```python
from build123d import *

# Parameters (mm, degrees)
SKETCH3_W           = 10.7
SKETCH3_H           = 10.7
BOSS_EXTRUDE2_DEPTH = 2.41
SKETCH5_R           = 1.25
BOSS_EXTRUDE3_DEPTH = 1.5875


with BuildPart() as part:
    # Sketch3 → Boss-Extrude2 (new body)
    with BuildSketch(Plane(origin=(0, 1.5875, 0), x_dir=(-1, 0, 0), z_dir=(0, 1, 0))):
        with Locations((-12.36, -20.96)):
            Rectangle(SKETCH3_W, SKETCH3_H)
    extrude(amount=BOSS_EXTRUDE2_DEPTH)

    # Sketch5 → Boss-Extrude3 (add)
    with BuildSketch(Plane.XZ.offset(-1.5875)):
        with Locations((16.36, -24.96)):
            Circle(SKETCH5_R)
        with Locations((12.36, -24.96)):
            Circle(SKETCH5_R)
        with Locations((8.36, -24.96)):
            Circle(SKETCH5_R)
        with Locations((16.36, -20.96)):
            Circle(SKETCH5_R)
        with Locations((12.36, -20.96)):
            Circle(SKETCH5_R)
        with Locations((8.36, -20.96)):
            Circle(SKETCH5_R)
        with Locations((16.36, -16.96)):
            Circle(SKETCH5_R)
        with Locations((12.36, -16.96)):
            Circle(SKETCH5_R)
        with Locations((8.36, -16.96)):
            Circle(SKETCH5_R)
    extrude(amount=BOSS_EXTRUDE3_DEPTH)


solid = part.part
```
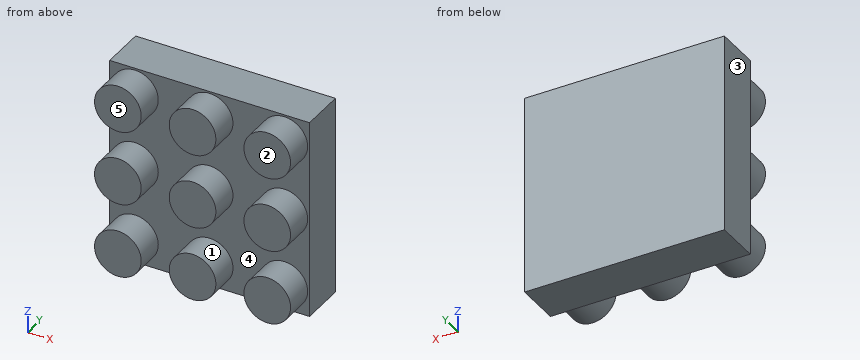
Part model, mm, in its own coordinate system. Face numbers are marked on the shaded views. A direction names the side the tool comes from. Round coordinates to 2 decimals unless told otherwise and drop trailing zeros. Write each loop counter-clockwise with the first axis right and the second up, starting at its lowest first coordinate (ties: lowest second). Pieces come first, ordered by that corner, then holes. Notation, with made-up numbers: M -14,64.25 L 4,64.25 A30 ccw 4,101.25 Z; hole C 67,65.5 d7. An arc over 180 degrees is marked long. Answer as CSV lines item,"result". Start each with the question number.
1) Band-saw the part on C-C (z = -23.5). List the corners of the cut face in (x, y).
2) Drop a flat-ended pin along its axis: pin 1 (2 mm diameter, centred on y = 0.5, z = -20, fed in from -X). Give the stop position or say it passes through.
3) Mould opens along X. For the marked faces 3, 4 and 5 say: +X half, -X half, draft (parallel to the pull), parting line (faces both ways), or undercut.
4) Drill centre lines: L1, parallel to X at y = 0.85, z = -21; L2, parallel to Z at x = 12, y = 1.35; L3, parallel to Z at x = 13, y = 0.8. Where is each one in solid material? Low to high.
5) Which spindle directions (+Z, -Z, +X, -X, +Y, -Y) get a long thin tool onto all of the face, cutting with end or side? Do the marked faces 1 and 2. Say none if no direction does.
6) Band-saw the part on A-A (x = 8.36). List the corners of the cut face in (y, z), then the cut area to 3 significant figures.
7) Band-saw the part on D-D (x = 14). List the corners of the cut face in (y, z).
8) Band-saw the part on B-B (z = -24.96). List the corners of the cut face in (x, y).
Worked out:
1,outline,"M 7.01,1.59 L 17.71,1.59 L 17.71,4 L 7.01,4 Z"
2,pin 1,"x = 7.11"
3,face 3,"-X half"
3,face 4,"undercut"
3,face 5,"draft"
4,L1,"7.11 to 9.61, 11.11 to 13.61, 15.11 to 17.61"
4,L2,"-26.16 to -23.76, -22.16 to -19.76, -18.16 to -15.76"
4,L3,"-26.03 to -23.89, -22.03 to -19.89, -18.03 to -15.89"
5,face 1,"-Y"
5,face 2,"+Z, -Z, +X, -X, -Y"
6,outline,"M 0,-26.21 L 1.59,-26.21 L 1.59,-26.31 L 4,-26.31 L 4,-15.61 L 1.59,-15.61 L 1.59,-15.71 L 0,-15.71 L 0,-18.21 L 1.59,-18.21 L 1.59,-19.71 L 0,-19.71 L 0,-22.21 L 1.59,-22.21 L 1.59,-23.71 L 0,-23.71 Z"
6,area,"37.7 mm²"
7,outline,"M 1.59,-26.31 L 4,-26.31 L 4,-15.61 L 1.59,-15.61 Z"
8,outline,"M 7.01,1.59 L 7.11,1.59 L 7.11,0 L 9.61,0 L 9.61,1.59 L 11.11,1.59 L 11.11,0 L 13.61,0 L 13.61,1.59 L 15.11,1.59 L 15.11,0 L 17.61,0 L 17.61,1.59 L 17.71,1.59 L 17.71,4 L 7.01,4 Z"
